Check sheet for the modelled part. Datum: model origin and axes. Units: mm. Face numbers are marked on the shaded views. Give positions to 0.01 mm unless a question says otherwise; leave off trailing zeros. Order: outer loops, then holes, each group sorted by start corner. A loop starts at its lowest first (then second) coordinate and runs counter-clockwise, first axis right, second up. Notation, with made-up numbers: (-39.5, 46) -> (17.5, 46) arc R17 cw to (17.5, 51) -> close; hole circle Ø3 at (74.5, 82.25). An arc over 180 degrees is marked (long way). Answer in a Markdown table with one row per item. Add a question column.
(1) Go/stop test with flat-tipped pins: pin 1 (1.5 mm diameter, centred on y = 6, z = 5, fed in from +X); pin 2 (3 mm diameter, centred on y = 7.5, z = 2, fed in from -X); pin 3 (2.5 mm diameter, centred on x = 3, y = 35, fed in from -Z); pin 4 (4.5 mm diameter, centred on y = 16.5, z = 6.5, fed in from +X). Record where each tip stops, or that it passes through.
(2) Cross-section at A-A (y = 25). State how many separate pieces and enclosed holes the cut face has, then the cut area to 3 significant figures.
(3) Thickness scan on L1, parallel to Y at x = 3, z = 7; L2, parallel to X at y = 7.5, z = 8.5; L3, parallel to Y at x = 14.7, z = 3.5. Record the ranges inside material, lowest first. Write a range as [from, to].
(4) Cross-section at C-C (x = 13). Record the cut outline in (y, z), then the cut area to 3 significant figures.
(5) Release check for a two-part mould opening along X. For the marked faces 1, 2 and 3 record: released by +X, released by -X, zero draft, split by the parting line, or undercut.
(6) Cross-section at D-D (y = 14). Record the cut outline in (x, z), then the cut area to 3 significant figures.
```python
from build123d import *

# Parameters (mm, degrees)
ESQUISSE1_W                  = 38
ESQUISSE1_H                  = 38
BOSS_EXTRU_1_DEPTH           = 9
ESQUISSE2_W                  = 14
ESQUISSE2_H                  = 38
ESQUISSE2_W_2                = 5.5
ENL_V_MAT_EXTRU_1_DEPTH      = 7.75
ESQUISSE3_R                  = 1.55
ENL_V_MAT_EXTRU_2_DEPTH      = 25
CONG_1_R                     = 3
CONG_2_R                     = 2
ESQUISSE9_R                  = 2.5
BOSS_EXTRU_2_DEPTH           = 2
ESQUISSE5_R                  = 1.55
ENL_V_MAT_EXTRU_4_DEPTH      = 8.75
ENL_V_MAT_EXTRU_4_DEPTH_BACK = 2.25
ESQUISSE10_W                 = 4
ESQUISSE10_H                 = 26
ENL_V_MAT_EXTRU_5_DEPTH      = 10
CONG_3_R                     = 1.5


with BuildPart() as part:
    # Esquisse1 → Boss.-Extru.1 (new body)
    with BuildSketch(Plane.XY):
        with Locations((19, 19)):
            Rectangle(ESQUISSE1_W, ESQUISSE1_H)
    extrude(amount=BOSS_EXTRU_1_DEPTH)

    # Esquisse2 → Enlèv. mat.-Extru.1 (cut)
    with BuildSketch(Plane(origin=(0, 0, 0), x_dir=(-1, 0, 0), z_dir=(0, 0, -1))):
        with Locations((-7, 19)):
            Rectangle(ESQUISSE2_W, ESQUISSE2_H)
        with Locations((-31, 19)):
            Rectangle(ESQUISSE2_W, ESQUISSE2_H)
        with Locations((-19, 19)):
            Rectangle(ESQUISSE2_W_2, ESQUISSE2_H)
    extrude(amount=-ENL_V_MAT_EXTRU_1_DEPTH, mode=Mode.SUBTRACT)

    # Esquisse3 → Enlèv. mat.-Extru.2 (cut, through all)
    with BuildSketch(Plane(origin=(24, 0, 0), x_dir=(0, 0, -1), z_dir=(1, 0, 0))):
        with Locations((-3.5, 10)):
            Circle(ESQUISSE3_R)
        with Locations((-3.5, 35)):
            Circle(ESQUISSE3_R)
        with Locations((-3.5, 25)):
            Circle(ESQUISSE3_R)
    extrude(amount=-ENL_V_MAT_EXTRU_2_DEPTH, mode=Mode.SUBTRACT)

    # Congé1
    cong_1_edges = [part.edges().sort_by_distance(p)[0] for p in [
        (0, 38, 8.375),
        (38, 38, 8.375),
        (38, 0, 8.375),
        (0, 0, 8.375),
    ]]
    fillet(cong_1_edges, radius=CONG_1_R)

    # Congé2
    cong_2_edges = [part.edges().sort_by_distance(p)[0] for p in [
        (22.875, 38, 0),
        (15.125, 38, 0),
        (15.125, 0, 0),
        (22.875, 0, 0),
    ]]
    fillet(cong_2_edges, radius=CONG_2_R)

    # Esquisse9 → Boss.-Extru.2 (add)
    with BuildSketch(Plane(origin=(0, 0, 7.75), x_dir=(-1, 0, 0), z_dir=(0, 0, -1))):
        with Locations((-35, 35)):
            Circle(ESQUISSE9_R)
        with Locations((-3, 35)):
            Circle(ESQUISSE9_R)
        with Locations((-3, 3)):
            Circle(ESQUISSE9_R)
        with Locations((-35, 3)):
            Circle(ESQUISSE9_R)
    extrude(amount=BOSS_EXTRU_2_DEPTH)

    # Esquisse5 → Enlèv. mat.-Extru.4 (cut, two sides)
    with BuildSketch(Plane(origin=(0, 0, 7.75), x_dir=(-1, 0, 0), z_dir=(0, 0, -1))) as enl_v_mat_extru_4_sk:
        with Locations((-35, 35)):
            Circle(ESQUISSE5_R)
        with Locations((-35, 3)):
            Circle(ESQUISSE5_R)
        with Locations((-3, 3)):
            Circle(ESQUISSE5_R)
        with Locations((-3, 35)):
            Circle(ESQUISSE5_R)
    extrude(amount=ENL_V_MAT_EXTRU_4_DEPTH, mode=Mode.SUBTRACT)
    extrude(enl_v_mat_extru_4_sk.sketch, amount=-ENL_V_MAT_EXTRU_4_DEPTH_BACK, mode=Mode.SUBTRACT)

    # Esquisse10 → Enlèv. mat.-Extru.5 (cut, through all)
    with BuildSketch(Plane.XY.offset(9)):
        with Locations((12, 19)):
            Rectangle(ESQUISSE10_W, ESQUISSE10_H)
        with Locations((5, 19)):
            Rectangle(ESQUISSE10_W, ESQUISSE10_H)
        with Locations((26, 19)):
            Rectangle(ESQUISSE10_W, ESQUISSE10_H)
        with Locations((33, 19)):
            Rectangle(ESQUISSE10_W, ESQUISSE10_H)
    extrude(amount=-ENL_V_MAT_EXTRU_5_DEPTH, mode=Mode.SUBTRACT)

    # Congé3
    cong_3_edges = [part.edges().sort_by_distance(p)[0] for p in [
        (3, 6, 8.375),
        (3, 32, 8.375),
        (7, 32, 8.375),
        (7, 6, 8.375),
        (24, 6, 8.375),
        (24, 32, 8.375),
        (28, 32, 8.375),
        (28, 6, 8.375),
        (35, 32, 8.375),
        (35, 6, 8.375),
        (31, 6, 8.375),
        (31, 32, 8.375),
        (14, 32, 8.375),
        (10, 6, 8.375),
        (10, 32, 8.375),
        (14, 6, 8.375),
    ]]
    fillet(cong_3_edges, radius=CONG_3_R)


solid = part.part
```
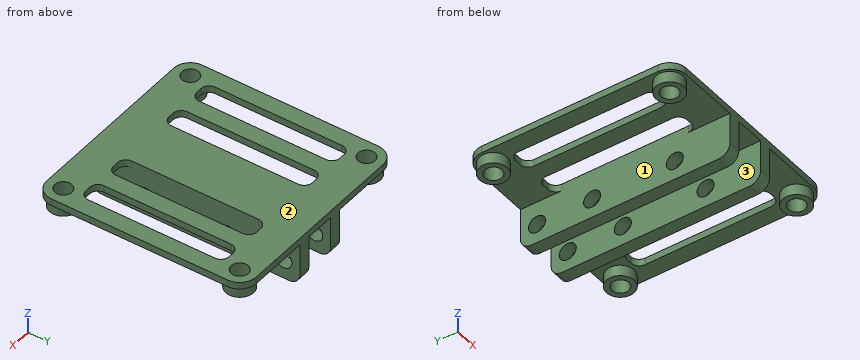
Answer below:
| question | item | result |
|---|---|---|
| 1 | pin 1 | stops at x = 24 |
| 1 | pin 2 | stops at x = 14 |
| 1 | pin 3 | passes through |
| 1 | pin 4 | stops at x = 38 |
| 2 | separate pieces | 7 |
| 2 | enclosed holes | 0 |
| 2 | area | 48.4 mm² |
| 3 | L1 | y = [0.5, 1.45], [4.55, 5.5], [32.5, 33.45], [36.55, 37.5] |
| 3 | L2 | x = [0, 3], [7, 10], [14, 24], [28, 31], [35, 38] |
| 3 | L3 | y = [0, 8.45], [11.55, 23.45], [26.55, 33.45], [36.55, 38] |
| 4 | outline | (0, 7.75) -> (6.09, 7.75) -> (6.09, 9) -> (0, 9) -> close; (31.91, 7.75) -> (38, 7.75) -> (38, 9) -> (31.91, 9) -> close |
| 4 | area | 15.2 mm² |
| 5 | face 1 | undercut |
| 5 | face 2 | zero draft |
| 5 | face 3 | undercut |
| 6 | outline | (0, 7.75) -> (3, 7.75) -> (3, 9) -> (0, 9) -> close; (7, 7.75) -> (10, 7.75) -> (10, 9) -> (7, 9) -> close; (14, 0) -> (16.25, 0) -> (16.25, 7.75) -> (21.75, 7.75) -> (21.75, 0) -> (24, 0) -> (24, 9) -> (14, 9) -> close; (28, 7.75) -> (31, 7.75) -> (31, 9) -> (28, 9) -> close; (35, 7.75) -> (38, 7.75) -> (38, 9) -> (35, 9) -> close |
| 6 | area | 62.4 mm² |
